Geometry check sheet. Reference: the model listing, model coordinates, mm. Coordinates: 2 decimals unless noted, no trailing zeros. Write each loop counter-clockwise with the first axis right and the second up, starting at its lowest first coordinate (ties: lowest second). Pieces come first, ordered by that corner, then holes. Notation, with made-up numbers: (21.5, 22.25) -> (38.5, 22.25) arc R18 cw to (38.5, 54.25) -> close; hole circle Ø11 at (58, 78). An arc over 180 degrees is marked (long way). Answer in a Markdown table with one row per item. Add a question column.
1. Cross-section at B-B on y = 26. Record the cut outline in (x, z), and give its area (3 significant figures).
2. Mould release check, pull along Y, two halves, no side actions. Record for faces 1 (the cylindrical face through (176.87, 287.43, -7.4)), 2 (the flat face through (129, 119, -15)), 3 (the flat face through (74, 0, -7)): pulls with the +Y half, pulls with the -Y half, needs draft (parallel to the pull), parting line crosses it, or undercut.
3. Scan lines: L1, parallel to X at y = 59.5, z = -12.5; L2, parallel to Y at x = 14, z = -6; L3, parallel to X at y = 25, z = -6.25. Record each from-to range of solid material in increasing order. Write a range as from..to.
4. Depth check by flat-ended pin: P1, Ø2, axis at x = 127, z = -10.5, coming from the +Y side; P2, Ø1.5, axis at x = 29.5, z = -7, coming from the +Y side; P3, Ø6, axis at x = 32, z = -4, coming from the -Y side; P4, Ø12, axis at x = 26.5, y = 73, coming from the -Z side. Enter the tip coordinate at first touch or a pass-through.
5. Cross-section at A-A on x = 189.5. Record the cut outline in (y, z), and give its area (3 significant figures).
```python
from build123d import *

# Parameters (mm, degrees)
BOSS_EXTRUDE1_DEPTH = 15
SKETCH3_R           = 11
CUT_EXTRUDE1_DEPTH  = 369.675083139


with BuildPart() as part:
    # Sketch2 → Boss-Extrude1 (new body)
    with BuildSketch(Plane.XY):
        with BuildLine():
            Line((0, 0), (150, 0))
            Line((150, 0), (213.766968501, 300))
            Line((213.766968501, 300), (163.766968501, 300))
            add(Edge.make_bspline(
                [(163.766968501, 300), (162.660354377, 183.828545376), (0, 40)],
                knots=[0, 0, 0, 0.298724745, 0.298724745, 0.298724745], degree=2))
            Line((0, 40), (0, 0))
        make_face()
    extrude(amount=-BOSS_EXTRUDE1_DEPTH)

    # Sketch3 → Cut-Extrude1 (cut, through all)
    with BuildSketch(Plane.XY):
        with Locations((184.979662991, 280)):
            Circle(SKETCH3_R)
    extrude(amount=-CUT_EXTRUDE1_DEPTH, mode=Mode.SUBTRACT)


solid = part.part
```
Results found:
| question | item | result |
|---|---|---|
| 1 | outline | (0, -15) -> (155.53, -15) -> (155.53, 0) -> (0, 0) -> close |
| 1 | area | 2,330 mm^2 |
| 2 | face 1 | undercut |
| 2 | face 2 | needs draft |
| 2 | face 3 | pulls with the -Y half |
| 3 | L1 | x = 21.45..162.65 |
| 3 | L2 | y = 0..52.6 |
| 3 | L3 | x = 0..155.31 |
| 4 | P1 | stops at y = 186.31 |
| 4 | P2 | stops at y = 67.85 |
| 4 | P3 | stops at y = 0 |
| 4 | P4 | passes through |
| 5 | outline | (185.83, -15) -> (269.97, -15) -> (269.97, 0) -> (185.83, 0) -> close; (290.03, -15) -> (300, -15) -> (300, 0) -> (290.03, 0) -> close |
| 5 | area | 1,410 mm^2 |
